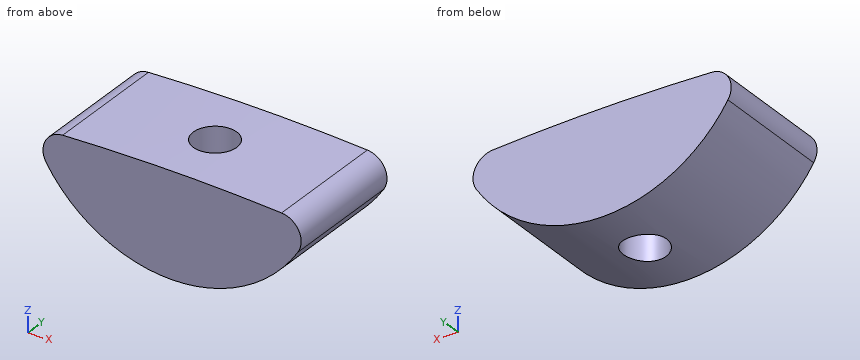
from build123d import *

# Parameters (mm, degrees)
BOSS_EXTRUDE1_DEPTH     = 4.826
SKETCH2_R               = 0.8509
CUT_EXTRUDE1_DEPTH      = 4.826
CUT_EXTRUDE1_DEPTH_BACK = 4.826


with BuildPart() as part:
    # Sketch1 → Boss-Extrude1 (new body)
    with BuildSketch(Plane(origin=(0, 0, 0), x_dir=(1, 0, 0), z_dir=(0, 1, 0))):
        with BuildLine():
            ThreePointArc((-4.285409449, -1.920000792), (0, -2.032), (4.285409449, -1.920000792))
            ThreePointArc((4.285409449, -1.920000792), (4.964968073, -1.480948711), (4.928136529, -0.672734574))
            ThreePointArc((4.928136529, -0.672734574), (0, 2.032), (-4.928136529, -0.672734574))
            ThreePointArc((-4.928136529, -0.672734574), (-4.964968073, -1.480948711), (-4.285409449, -1.920000792))
        make_face()
    extrude(amount=BOSS_EXTRUDE1_DEPTH)

    # Sketch2 → Cut-Extrude1 (cut, two sides)
    with BuildSketch(Plane.XY) as cut_extrude1_sk:
        with Locations((0, 2.413)):
            Circle(SKETCH2_R)
    extrude(amount=CUT_EXTRUDE1_DEPTH, mode=Mode.SUBTRACT)
    extrude(cut_extrude1_sk.sketch, amount=-CUT_EXTRUDE1_DEPTH_BACK, mode=Mode.SUBTRACT)


solid = part.part
Verification items for the finished model (mm, model axes). Coordinates: 2 decimals unless noted, no trailing zeros. Write each loop counter-clockwise with the first axis right and the second up, starting at its lowest first coordinate (ties: lowest second). Pieces come first, ordered by that corner, then holes. Notation, with made-up numbers: (-34, -21) - (-15, -21) arc R19 cw to (-15, -15) - close; hole circle Ø2 at (13, 47). An arc over 180 degrees is marked (long way). Answer as a JSON object with one key per item and string values.
(1) Cross-section at D-D on y = 0.9. Record the cut outline in (x, z), plus the area to 3 significant figures.
Report:
{"outline": "(-4.93, 0.67) arc R5.84 ccw to (4.93, 0.67) arc R0.81 ccw to (4.29, 1.92) arc R82.04 ccw to (-4.29, 1.92) arc R0.81 ccw to start", "area": "31.7 mm^2"}
(2) Thickness scan on line 1 along Y through (x, z) = (0, 1.15); line 2 along X through (y, z) = (1.75, -0.75); line 3 along X through (y, z) = (1.65, -1.45). Record the ranges inside material, lowest first.
Report:
{"line 1": "0 to 1.56, 3.26 to 4.83", "line 2": "-3.65 to -0.53, 0.53 to 3.65", "line 3": "-2.54 to -0.38, 0.38 to 2.54"}
(3) Cross-section at A-A on x = 0. Record the cut outline in (y, z).
Report:
{"outline": "(0, -2.03) - (1.56, -2.03) - (1.56, 2.03) - (0, 2.03) - close; (3.26, -2.03) - (4.83, -2.03) - (4.83, 2.03) - (3.26, 2.03) - close"}
(4) Cross-section at B-B on y = 2.25. Record the cut outline in (x, z), plus the area to 3 significant figures.
Report:
{"outline": "(-4.93, 0.67) arc R5.84 ccw to (-0.84, -1.97) - (-0.84, 2.03) arc R82.04 ccw to (-4.29, 1.92) arc R0.81 ccw to start; (0.84, -1.97) arc R5.84 ccw to (4.93, 0.67) arc R0.81 ccw to (4.29, 1.92) arc R82.04 ccw to (0.84, 2.03) - close", "area": "25.0 mm^2"}
(5) Cross-section at C-C on z = -1.7. Record the cut outline in (x, y), plus the area to 3 significant figures.
Report:
{"outline": "(-1.94, 0) - (1.94, 0) - (1.94, 4.83) - (-1.94, 4.83) - close; hole circle Ø1.7 at (0, 2.41)", "area": "16.5 mm^2"}
